```python
from build123d import *

# Parameters (mm, degrees)
SKETCH3_R      = 6
EXTRUDE1_DEPTH = 8.9375
SKETCH4_R      = 1
SKETCH4_R_2    = 1.25
EXTRUDE2_DEPTH = 8.9375


with BuildPart() as part:
    # Sketch1 → Revolve1 (revolve)
    with BuildSketch(Plane.XY):
        with BuildLine():
            Line((0, 0), (7.9375, 0))
            Line((7.9375, 0), (7.9375, 14))
            Line((7.9375, 14), (7.9375, 17.175))
            Line((7.9375, 17.175), (7.9375, 18.365625))
            Line((7.9375, 18.365625), (6.746875, 18.365625))
            Line((6.746875, 18.365625), (6.746875, 17.175))
            ThreePointArc((6.746875, 17.175), (3.96875, 14.396875), (1.190625, 17.175))
            Line((1.190625, 17.175), (1.190625, 18.365625))
            Line((1.190625, 18.365625), (0, 18.365625))
            Line((0, 18.365625), (0, 17.175))
            Line((0, 17.175), (0, 14))
            Line((0, 14), (0, 0))
        make_face()
    revolve(axis=Axis((0, 0, 0), (1, 0, 0)))

    # Sketch3 → Extrude1 (cut, through all)
    with BuildSketch(Plane(origin=(7.9375, 0, 0), x_dir=(0, 0, -1), z_dir=(1, 0, 0))):
        Circle(SKETCH3_R)
    extrude(amount=-EXTRUDE1_DEPTH, mode=Mode.SUBTRACT)

    # Sketch4 → Extrude2 (cut, through all)
    with BuildSketch(Plane(origin=(7.9375, 0, 0), x_dir=(0, 0, -1), z_dir=(1, 0, 0))):
        with Locations((0, 11)):
            Circle(SKETCH4_R)
        with Locations((-4.381841494, 10.089572098)):
            Circle(SKETCH4_R_2)
        with Locations((4.381841494, 10.089572098)):
            Circle(SKETCH4_R_2)
        with Locations((10.089572098, -4.381841494)):
            Circle(SKETCH4_R_2)
        with Locations((11, 0)):
            Circle(SKETCH4_R)
        with Locations((10.089572098, 4.381841494)):
            Circle(SKETCH4_R_2)
        with Locations((-4.381841494, -10.089572098)):
            Circle(SKETCH4_R_2)
        with Locations((0, -11)):
            Circle(SKETCH4_R)
        with Locations((4.381841494, -10.089572098)):
            Circle(SKETCH4_R_2)
        with Locations((-10.089572098, 4.381841494)):
            Circle(SKETCH4_R_2)
        with Locations((-11, 0)):
            Circle(SKETCH4_R)
        with Locations((-10.089572098, -4.381841494)):
            Circle(SKETCH4_R_2)
    extrude(amount=-EXTRUDE2_DEPTH, mode=Mode.SUBTRACT)


solid = part.part
```
Verification items for the finished model (mm, model axes). A direction names the side the tool comes from. Give positions to 0.01 mm unless a question says otherwise; leave off trailing zeros. Write each loop counter-clockwise with the first axis right and the second up, starting at its lowest first coordinate (ties: lowest second). Pieces come first, ordered by that corner, then holes. Notation, with made-up numbers: (-13, 64.25) - (36, 64.25) arc R23 cw to (36, 84.25) - close; hole circle Ø1 at (58, 38). An arc over 180 degrees is marked (long way). Put each result on its own line as item: value.
Q1. Mould release check, pull along X, two halves, no side actions. Record for faces 3 (the face through (4, 10, 0)), 4 (the face through (1.191, -14, -11)), 5 (the face through (7.938, 0, -8)): released by +X, released by -X, zero draft, split by the parting line, or undercut.
Result:
face 3: zero draft
face 4: undercut
face 5: released by +X
Q2. Section check C-C on x = 2.25. Count the separate pieces of the cut face and the enclosed holes in it, and give its area (3 significant figures).
Result:
separate pieces: 1
enclosed holes: 13
area: 541 mm2
Q3. Scan lines: probe 1 along X at (y, z) = (14.5, 10.5); probe 2 along Z at (x, y) = (6.5, 4); probe 3 along Y at (x, z) = (1.5, 9). Record each from-to range of solid material in increasing order. Write a range as from..to.
Result:
probe 1: 0..1.19, 6.75..7.94
probe 2: -15.52..-11.28, -8.9..-4.47, 4.47..8.9, 11.28..15.52
probe 3: -13.11..-4.99, -3.77..3.77, 4.99..13.11
Q4. Section check A-A on y = 0. Record the cut outline in (x, z) (1 decimal).
Result:
outline: (0, -18.4) - (1.2, -18.4) - (1.2, -17.2) arc R2.8 cw to (6.7, -17.2) - (6.7, -18.4) - (7.9, -18.4) - (7.9, -12) - (0, -12) - close; (0, -10) - (7.9, -10) - (7.9, -6) - (0, -6) - close; (0, 6) - (7.9, 6) - (7.9, 10) - (0, 10) - close; (0, 12) - (7.9, 12) - (7.9, 18.4) - (6.7, 18.4) - (6.7, 17.2) arc R2.8 cw to (1.2, 17.2) - (1.2, 18.4) - (0, 18.4) - close
Q5. Set-up check for faces 1 (the face through (4.024, -3.328, 9.418)), 2 (the face through (6.747, 14, -11)): record each of +Z, -Z, +X, -X, +Y, -Y from which the full face is reachable in a straight line by a thin tool's end or side.
Result:
face 1: +X, -X
face 2: none
Q6. Depth check by flat-ended pin: P1, Ø4, axis at y = -4.38, z = 10.09, coming from the -X side; P2, Ø1, axis at x = 2, z = -2.5, coming from the +Y side; P3, Ø3, axis at x = 7, y = -9.5, coming from the -Z side. Enter the tip coordinate at first touch or a pass-through.
Result:
P1: x = 0
P2: y = 15.71
P3: z = -16.53
